```python
from build123d import *

# Parameters (mm, degrees)
SKETCH001_W             = 13
SKETCH001_H             = 26
SKETCH001_W_2           = 3
SKETCH001_H_2           = 16
PAD001_DEPTH            = 66
BOX_W                   = 16
BOX_H                   = 7
BOX_DEPTH               = 8
BOX001_W                = 15
BOX001_H                = 5
BOX001_DEPTH            = 59
BOX002_W                = 4
BOX002_H                = 5
BOX002_DEPTH            = 59
BODY001_PLACEMENT_ANGLE = 180


with BuildPart() as part:
    # Sketch001 → Pad001 (new body)
    with BuildSketch(Plane.XY):
        with Locations((1, 0)):
            Rectangle(SKETCH001_W, SKETCH001_H)
        with Locations((1, 0)):
            Rectangle(SKETCH001_W_2, SKETCH001_H_2, mode=Mode.SUBTRACT)
    extrude(amount=PAD001_DEPTH)

    # Box → Box (cut)
    with BuildSketch(Plane(origin=(0, -8, 0), x_dir=(0, 1, 0), z_dir=(1, 0, 0))):
        with Locations((8, 3.5)):
            Rectangle(BOX_W, BOX_H)
    extrude(amount=BOX_DEPTH, mode=Mode.SUBTRACT)

    # Box001 → Box001 (join)
    with BuildSketch(Plane(origin=(-5.5, 8, 5), x_dir=(0, 1, 0), z_dir=(1, 0, 0))):
        with Locations((7.5, 2.5)):
            Rectangle(BOX001_W, BOX001_H)
    extrude(amount=BOX001_DEPTH)

    # Box002 → Box002 (join)
    with BuildSketch(Plane(origin=(-5.5, 19, 0), x_dir=(0, 1, 0), z_dir=(1, 0, 0))):
        with Locations((2, 2.5)):
            Rectangle(BOX002_W, BOX002_H)
    extrude(amount=BOX002_DEPTH)


with BuildPart() as part_1:
    # Body001 placement: moved
    add(part.part.rotate(Axis((0, 0, 0), (1, 0, 0)), BODY001_PLACEMENT_ANGLE))


solid = part_1.part
```
The model under review builds one solid part; all positions refer to its coordinate system, in mm. A direction names the side the tool comes from. Round coordinates to 2 decimals unless told otherwise and drop trailing zeros. Loops run counter-clockwise (first coordinate to the right, second up) from the corner with the lowest first, then second, coordinate; pieces in that order, holes last.
Item 1: Mouldability with a two-part tool opening along X and no side actions: class faces 1 (the face through (7.5, -10, -2)), 2 (the face through (24, -13, -5)), 3 (the face through (2, 8, -25)) as released by +X, released by -X, zero draft, split by the parting line, or undercut.
Determined:
face 1: released by +X
face 2: zero draft
face 3: undercut
Item 2: Clearance check with flat-ended pins moving along their axes: pin 1 Ø2 at (x, y) = (24, -15.5) entering from +Z; pin 2 Ø4 at (x, z) = (23, -3.5) entering from +Y; pin 3 Ø9 at (x, z) = (3, -46.5) entering from -Y. State where each tip first meets the part, or that it passes through.
Determined:
pin 1: stops at z = -5
pin 2: stops at y = -8
pin 3: stops at y = -13
Item 3: Take a section at B-B (z = -50). Write out the cut boundary in (x, y).
Determined:
outline: (-5.5, -13) - (7.5, -13) - (7.5, 13) - (-5.5, 13) - close; hole (-0.5, -8) - (2.5, -8) - (2.5, 8) - (-0.5, 8) - close
Item 4: For faces 4 (the face through (5, 0, -7)), 5 (the face through (2.5, 0, -36)), 6 (the face through (1, -13, -38)), 7 (the face through (24, -21, 0)), 8 (the face through (1, -13, -2)), list the 3-axis set-ups (+Z, -Z, +X, -X, +Y, -Y) from which the entire face can be reached by the end or side of a thin tool; tool diameter is ignored.
Determined:
face 4: +Z, +X
face 5: +Z, -Z
face 6: -Z, +X, -X, -Y
face 7: +Z, +X, -X, +Y, -Y
face 8: +Z, +X, -X
Item 5: Take a section at A-A (y = -5.5). Write out the cut boundary in (x, z), then the cut area to 3 significant figures.
Determined:
outline: (-5.5, -66) - (-0.5, -66) - (-0.5, 0) - (-5.5, 0) - close; (2.5, -66) - (7.5, -66) - (7.5, -7) - (2.5, -7) - close
area: 625 mm2
Item 6: Take a section at D-D (y = 10). Write out the cut boundary in (x, z).
Determined:
outline: (-5.5, -66) - (7.5, -66) - (7.5, 0) - (-5.5, 0) - close
Item 7: For line 1 (X direction, y = -2.5, z = -45); line 2 (Y direction, x = 1.5, z = -56); line 3 (Y direction, x = -2, z = -3), list the stretches that pass through material, from the lowest coordinate up.
Determined:
line 1: x = -5.5 to -0.5, 2.5 to 7.5
line 2: y = -13 to -8, 8 to 13
line 3: y = -23 to -19, -13 to 13
Item 8: Take a section at C-C (x = 48.5). Write out the cut boundary in (y, z).
Determined:
outline: (-23, -10) - (-8, -10) - (-8, -5) - (-19, -5) - (-19, 0) - (-23, 0) - close
